For this review, take the finished solid that the model builds, in its own axes (mm). Face numbers are marked on the shaded views. A direction names the side the tool comes from. Give positions to 0.01 mm unless a question says otherwise; leave off trailing zeros. Write each loop counter-clockwise with the first axis right and the second up, starting at its lowest first coordinate (ties: lowest second). Pieces come first, ordered by that corner, then holes. Notation, with made-up numbers: (48.25, -26) -> (72.25, -26) arc R17 ccw to (72.25, 3) -> close; hole circle Ø7 at (15.5, 45.25). An arc over 180 degrees is marked (long way). Answer as CSV lines item,"result".
```python
from build123d import *

# Parameters (mm, degrees)
SKETCH1_W           = 43
SKETCH1_H           = 21.4
BOSS_EXTRUDE1_DEPTH = 2
SKETCH2_R           = 1.45
CUT_EXTRUDE1_DEPTH  = 25.098547674
SKETCH3_W           = 10
SKETCH3_H           = 4
BOSS_EXTRUDE2_DEPTH = 10
SKETCH4_R           = 1
BOSS_EXTRUDE3_DEPTH = 1.7
SKETCH5_W           = 0.7
SKETCH5_H           = 1.5
BOSS_EXTRUDE4_DEPTH = 0.75


with BuildPart() as part:
    # Sketch1 → Boss-Extrude1 (new body)
    with BuildSketch(Plane(origin=(0, 0, 0), x_dir=(1, 0, 0), z_dir=(0, 1, 0))):
        Rectangle(SKETCH1_W, SKETCH1_H)
    extrude(amount=BOSS_EXTRUDE1_DEPTH)

    # Sketch2 → Cut-Extrude1 (cut, through all)
    with BuildSketch(Plane(origin=(0, 2, 0), x_dir=(1, 0, 0), z_dir=(0, 1, 0))):
        with Locations(Location((-15.05, 8.05, 0), (0, 0, 270))):
            Circle(SKETCH2_R)
        with Locations(Location((15.05, -8.05, 0), (0, 0, 270))):
            Circle(SKETCH2_R)
    extrude(amount=-CUT_EXTRUDE1_DEPTH, mode=Mode.SUBTRACT)

    # Sketch3 → Boss-Extrude2 (add)
    with BuildSketch(Plane(origin=(0, 2, 0), x_dir=(1, 0, 0), z_dir=(0, 1, 0))):
        with Locations((-7.25, -7.7)):
            Rectangle(SKETCH3_W, SKETCH3_H)
    extrude(amount=BOSS_EXTRUDE2_DEPTH)

    # Sketch4 → Boss-Extrude3 (add)
    with BuildSketch(Plane(origin=(0, 12, 0), x_dir=(1, 0, 0), z_dir=(0, 1, 0))):
        with Locations(Location((-3.25, -8.7, 0), (0, 0, 270))):
            Circle(SKETCH4_R)
    extrude(amount=BOSS_EXTRUDE3_DEPTH)

    # Sketch5 → Boss-Extrude4 (add)
    with BuildSketch(Plane(origin=(0, 2, 0), x_dir=(1, 0, 0), z_dir=(0, 1, 0))):
        with Locations((-16, -8.5)):
            Rectangle(SKETCH5_W, SKETCH5_H)
    extrude(amount=BOSS_EXTRUDE4_DEPTH)


solid = part.part
```
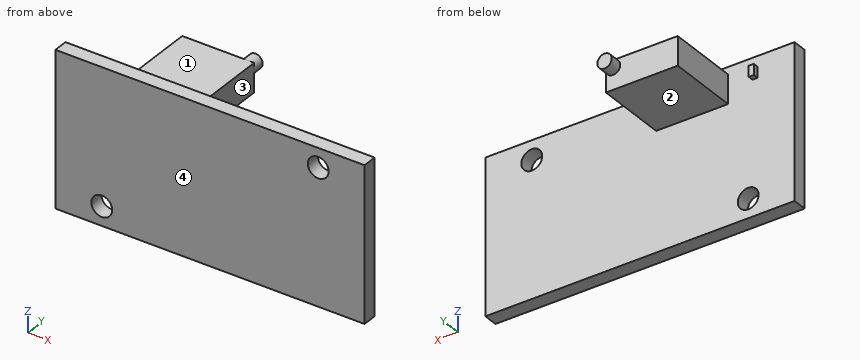
Q1. Add section A-A (x = 15.05). Write out the cut boundary in (y, z), plus the area to 3 significant figures.
Answer block:
outline,"(0, -10.7) -> (2, -10.7) -> (2, 6.6) -> (0, 6.6) -> close; (0, 9.5) -> (2, 9.5) -> (2, 10.7) -> (0, 10.7) -> close"
area,"37.0 mm2"
Q2. For the marked faces 1, 2, 3 and 4, list the 3-axis set-ups (+Z, -Z, +X, -X, +Y, -Y) from which the entire face can be reached by the end or side of a thin tool; tool diameter is ignored.
Answer block:
face 1,"+Z, +X, -X, +Y"
face 2,"-Z, +X, -X, +Y"
face 3,"+Z, -Z, +X, +Y"
face 4,"+Z, -Z, +X, -X, -Y"
Q3. Clearance check with flat-ended pins moving along their axes: pin 1 (0.8 mm diameter, centred on x = -16, y = 2.5, fed in from +Z); pin 2 (3 mm diameter, centred on x = -6, y = 4, fed in from -Z); pin 3 (3 mm diameter, centred on x = -9.5, z = 7, fed in from +Y). State where each tip first meets the part, or that it passes through.
Answer block:
pin 1,"stops at z = 9.25"
pin 2,"stops at z = 5.7"
pin 3,"stops at y = 12"
Q4. Add section D-D (x = 2.5). Write out the cut boundary in (y, z), plus the area to 3 significant figures.
Answer block:
outline,"(0, -10.7) -> (2, -10.7) -> (2, 10.7) -> (0, 10.7) -> close"
area,"42.8 mm2"
Q5. Add section B-B (z = -8.05). Write out the cut boundary in (x, y), plus the area to 3 significant figures.
Answer block:
outline,"(-21.5, 0) -> (-16.5, 0) -> (-16.5, 2) -> (-21.5, 2) -> close; (-13.6, 0) -> (21.5, 0) -> (21.5, 2) -> (-13.6, 2) -> close"
area,"80.2 mm2"
Q6. Add section C-C (y = 7). Write out the cut boundary in (x, z).
Answer block:
outline,"(-12.25, 5.7) -> (-2.25, 5.7) -> (-2.25, 9.7) -> (-12.25, 9.7) -> close"
Q7. To check wall thickness, follow probe 1 along X at (y, z) = (1.5, 8.05); probe 2 along Y at (x, z) = (-4, 6); probe 3 along X at (y, z) = (10.75, 7). State the ranges of each line that lie inside material, in increasing order. Write a range as [from, to].
Answer block:
probe 1,"x = [-21.5, 13.6], [16.5, 21.5]"
probe 2,"y = [0, 12]"
probe 3,"x = [-12.25, -2.25]"
